Build history of the part. All positions in model axes, mm. A direction names the side the tool comes from. Round coordinates to 2 decimals unless told otherwise and drop trailing zeros. Order: outer loops, then holes, each group sorted by start corner. A loop starts at its lowest first (then second) coordinate and runs counter-clockwise, first axis right, second up. Notation, with made-up numbers: (41, -25.75) -> (90, -25.75) arc R15 cw to (90, -11.75) -> close; hole circle Ø2 at (54.25, -28). An arc over 180 degrees is marked (long way). Use a Markdown table: item, result. Add a question column.
Item 1: 3-axis set-ups, long thin cutter, end or side, ignore diameter. For faces 1 (the face through (6, -14, 2)), 2 (the face through (0, 0, -1)), 3 (the face through (-0.28, 14.53, 3.54)): which of +Z, -Z, +X, -X, +Y, -Y reach the whole face in a straight line?
Item 2: Two-plate mould, pull along Y, no slides. Class faces 4 (the face through (-6, -14, 2)), 5 (the face through (0, 0, 0)), 6 (the face through (6, 14, 2)): released by +Y, released by -Y, zero draft, split by the parting line, or undercut.
Item 3: Slice it at B-B, the plane y = -7.5. Give the cut face in (x, z), plus the area to 3 significant figures.
Item 4: Slice it at A-A, the plane x = 4. Give the cut face in (y, z), plus the area to 3 significant figures.
Item 5: Slice it at D-D, the plane y = 12.5. Give the cut face in (x, z).
Item 6: Pin check, flat tips, straight feed: pin 1 (2 mm diameter, centred on x = -5.5, z = 4, fed in from -Y); pin 2 (2 mm diameter, centred on x = -7.5, z = 3.5, fed in from +Y); pin 3 (3 mm diameter, centred on x = -3, z = 4.5, fed in from +Y); pin 4 (1.4 mm diameter, centred on x = 0, y = -14, fed in from +Z). Stop position of each tip, or through.
Item 7: Probe L1, parallel to Y at x = 0, z = 2.25; L2, parallel to Y at x = -7.75, z = 4; L3, parallel to X at y = 3.75, z = 4.5. List the from-to ranges inside material, lowest first.
Item 8: Slice it at C-C, the plane z = 1.5. State how many separate pieces and enclosed holes the cut face has, plus the area to 3 significant figures.
Autodesk Fusion 360 part; units mm, degrees
sketch "Boceto1" plane through (0, 0, 0) normal (0, 0, 1) x (1, 0, 0)
  line L0 (10, -14) -> (-10, -14)
  line L1 (-10, -14) -> (-10, 14)
  line L2 (-10, 14) -> (10, 14)
  line L3 (10, 14) -> (10, -14)
  line L4 (10, -14) -> (-10, 14) construction
  line L5 (-10, -14) -> (10, 14) construction
  line L6 (9, -13) -> (-9, -13)
  line L7 (-9, -13) -> (-9, 13)
  line L8 (-9, 13) -> (9, 13)
  line L9 (9, 13) -> (9, -13)
  line L10 (9, -13) -> (-9, 13) construction
  line L11 (-9, -13) -> (9, 13) construction
  dimension "d1" = 20
  dimension "d2" = 28
  dimension "d3" = 18
  dimension "d4" = 26
extrude "Extruir1" add sketch "Boceto1" against normal blind 1 contours L0 L1 L2 L3 | L6 L7 L8 L9
extrude "Extruir2" add sketch "Boceto1" along normal blind 6
sketch "Boceto2" plane through (10, 0, 0) normal (1, 0, 0) x (0, 1, 0)
  line L0 (-14, 6) -> (-14, -1)
  line L1 (-14, -1) -> (14, -1)
  line L2 (14, -1) -> (14, 6)
  line L3 (14, 6) -> (-14, 6)
  line L4 (13, 6) -> (-13, 6)
  line L5 (-13, 6) -> (13, 6)
  line L6 (14, 6) -> (-14, 6)
  line L7 (-14, 6) -> (14, 6)
  line L8 (-13, 0) -> (13, 0)
  line L9 (13, 0) -> (13, 6)
  line L10 (13, 6) -> (-13, 6)
  line L11 (-13, 6) -> (-13, 0)
  line L12 (-13, 0) -> (-3, 0)
  line L13 (-3, 0) -> (-2.997, 6)
  line L14 (-13, 6) -> (-2.997, 6)
  line L15 (-13, 0) -> (-13, 2.5)
  line L16 (-13, 2.5) -> (-2.9987, 2.4949)
  line L17 (-2.9987, 2.4949) -> (-3, 0)
  dimension "d9" = 10
  dimension "d12" = 2.5
extrude "Extruir3" cut sketch "Boceto2" against normal blind 28 contours L8 L11 L12 L13 L15 L16 L17
sketch "Boceto3" plane through (0, 0, 6) normal (0, 0, 1) x (-1, 0, 0)
  line L0 (9, -13) -> (-9, -13)
  line L1 (-9, -13) -> (-9, 13)
  line L2 (-9, 13) -> (9, 13)
  line L3 (9, 13) -> (9, -13)
  line L4 (-10, -14) -> (10, -14)
  line L5 (10, -14) -> (10, 14)
  line L6 (10, 14) -> (-10, 14)
  line L7 (-10, 14) -> (-10, -14)
  line L8 (0, -14) -> (2, -14) construction
  ellipse E0 centre (0, -14) end of major axis (2, -14) minor radius 1
  line L9 (0, -15) -> (0, -13) construction
  line L10 (0, 14) -> (2, 14) construction
  ellipse E1 centre (0, 14) end of major axis (2, 14) minor radius 1
  line L11 (-2, 14) -> (2, 14) construction
  line L12 (0, 13) -> (0, 15) construction
  circle A0 centre (0, 14) radius 0.6
  circle A1 centre (0, -14) radius 0.6
  dimension "d15" = 2
  dimension "d17" = 2
  dimension "d18" = 2
  dimension "d19" = 2
  dimension "d20" = 1.2
  dimension "d21" = 1.2
extrude "Extruir4" add sketch "Boceto3" against normal blind 7 contours L4 E0 A1 | L4 A1 | L6 E1 A0 | L6 A0 picked at (-1.4687, -14.1432) picked at (-0.0731, -14.1862) picked at (1.4687, 14.1432) picked at (0.1247, 14.1564)
extrude "Extruir5" cut sketch "Boceto3" against normal blind 5 contours L4 A1 | L4 A1 | L6 A0 | L6 A0
Check sheet entries:
| question | item | result |
|---|---|---|
| 1 | face 1 | +Z, -Z, +X, -Y |
| 1 | face 2 | -Z, +X, -X, +Y, -Y |
| 1 | face 3 | +Z |
| 2 | face 4 | released by -Y |
| 2 | face 5 | undercut |
| 2 | face 6 | released by +Y |
| 3 | outline | (-10, -1) -> (10, -1) -> (10, 0) -> (-10, 0) -> close; (-10, 2.5) -> (-9, 2.5) -> (-9, 6) -> (-10, 6) -> close; (9, 2.5) -> (10, 2.5) -> (10, 6) -> (9, 6) -> close |
| 3 | area | 27.0 mm2 |
| 4 | outline | (-14, -1) -> (14, -1) -> (14, 6) -> (13, 6) -> (13, 0) -> (-13, 0) -> (-13, 6) -> (-14, 6) -> close |
| 4 | area | 40.0 mm2 |
| 5 | outline | (-10, -1) -> (10, -1) -> (10, 6) -> (9, 6) -> (9, 0) -> (-9, 0) -> (-9, 6) -> (-10, 6) -> close |
| 6 | pin 1 | y = -14 |
| 6 | pin 2 | y = 14 |
| 6 | pin 3 | y = 14.66 |
| 6 | pin 4 | z = 6 |
| 7 | L1 | -15 to -14.6, -13.4 to -13, 13 to 13.4, 14.6 to 15 |
| 7 | L2 | -14 to -13, 13 to 14 |
| 7 | L3 | -10 to -9, 9 to 10 |
| 8 | separate pieces | 2 |
| 8 | enclosed holes | 2 |
| 8 | area | 76.0 mm2 |
